Autodesk Inventor part; units mm, degrees
ref_plane "Arbeitsebene1" through (0, 5.7, 0) normal (0, 1, 0) x (1, 0, 0)
ref_plane "YZ Plane" through (0, 0, 0) normal (1, 0, 0) x (0, 1, 0)
ref_plane "XZ Plane" through (0, 0, 0) normal (0, 1, 0) x (-1, 0, 0)
sketch "Skizze2" plane through (0, 0, 0) normal (0, 1, 0) x (-1, 0, 0)
  line L0 (0, 0) -> (2.4, 0)
  line L1 (2.4, 0) -> (2.4, -5)
  line L2 (2.4, -5) -> (0, -5)
  line L3 (0, -5) -> (0, 0)
  dimension "d0" = 2.4
  dimension "d1" = 5
extrude "Extrusion1" add sketch "Skizze2" along normal blind 6.3
sketch "Skizze3" plane through (0, 0, 0) normal (0, -1, 0) x (1, 0, 0)
  line L0 (-0.9, -3.47) -> (-1.5, -3.47)
  line L1 (-1.5, -3.47) -> (-1.5, -4.07)
  line L2 (-1.5, -4.07) -> (-0.9, -4.07)
  line L3 (-0.9, -4.07) -> (-0.9, -3.47)
  line L4 (-0.9, -0.93) -> (-1.5, -0.93)
  line L5 (-1.5, -0.93) -> (-1.5, -1.53)
  line L6 (-1.5, -1.53) -> (-0.9, -1.53)
  line L7 (-0.9, -1.53) -> (-0.9, -0.93)
  line L8 (-2.4, -5) -> (0, -5)
  line L9 (-2.4, 0) -> (-2.4, -5)
  point P0 (0, 0)
  dimension "d4" = 0.6
  dimension "d5" = 0.6
  dimension "d6" = 0.6
  dimension "d7" = 0.6
  dimension "d8" = 2.54
  dimension "d9" = 0.93
  dimension "d10" = 0.9
  dimension "d11" = 0.9
sketch "Skizze5" plane through (0, 0, 0) normal (0, -1, 0) x (1, 0, 0)
  line L0 (-0.5, -0.5) -> (-1.9, -0.5)
  line L1 (-1.9, -0.5) -> (-1.9, -4.5)
  line L2 (-1.9, -4.5) -> (-0.5, -4.5)
  line L3 (-0.5, -4.5) -> (-0.5, -0.5)
  line L4 (-2.4, 0) -> (-2.4, -5)
  line L5 (0, -5) -> (-2.4, -5)
  point P0 (0, 0)
  dimension "d15" = 1.4
  dimension "d16" = 4
  dimension "d17" = 0.5
  dimension "d18" = 0.5
extrude "Extrusion2" cut sketch "Skizze5" against normal blind 0.2
extrude "Extrusion3" cut sketch "Skizze3" against normal blind 6
ref_plane "Arbeitsebene1" through (0, 5.7, 0) normal (0, 1, 0) x (1, 0, 0)
sketch "Skizze6" plane through (0, 5.7, 0) normal (0, 1, 0) x (1, 0, 0)
  line L0 (1, -1) -> (-3, -1)
  line L1 (-3, -1) -> (-3, 6)
  line L2 (-3, 6) -> (1, 6)
  line L3 (1, 6) -> (1, -1)
  line L4 (-0.1, 4.9) -> (-2.3, 4.9)
  line L5 (-2.3, 4.9) -> (-2.3, 0.1)
  line L6 (-2.3, 0.1) -> (-0.1, 0.1)
  line L7 (-0.1, 0.1) -> (-0.1, 4.9)
  line L8 (0, 5) -> (-2.4, 5)
  line L9 (0, 0) -> (0, 5)
  line L10 (0, 0) -> (-2.4, 0)
  line L11 (-2.4, 5) -> (-2.4, 0)
  dimension "d24" = 0.1
  dimension "d25" = 0.1
  dimension "d26" = 0.1
  dimension "d27" = 0.1
extrude "Extrusion5" cut sketch "Skizze6" against normal blind 0.6 contours L0 L1 L2 L3 | L9 L10 L11 L8
sketch "Skizze7" plane through (0, 0.2, 0) normal (0, -1, 0) x (1, 0, 0)
  line L0 (-0.5, -2.004) -> (-1.5, -2.004)
  line L1 (-1.5, -2.004) -> (-1.5, -2.996)
  line L2 (-1.5, -2.996) -> (-0.5, -2.996)
  line L3 (-0.5, -2.996) -> (-0.5, -2.004)
  line L4 (-1.5, -3.47) -> (-0.9, -3.47)
  line L5 (-0.9, -1.53) -> (-1.5, -1.53)
  line L6 (-0.5, -0.5) -> (-0.5, -4.5)
  line L7 (-1.5, -1.53) -> (-1.5, -0.93)
  line L8 (-1.5, -2.004) -> (-1.217, -2.004)
  line L9 (-1.217, -2.004) -> (-1.217, -1.53)
  line L10 (-1.217, -1.53) -> (-1.5, -1.53)
  line L11 (-1.5, -1.53) -> (-1.5, -2.004)
  line L12 (-1.5, -3.47) -> (-0.9, -3.47)
  line L13 (-1.5, -2.996) -> (-1.217, -2.996)
  line L14 (-1.217, -2.996) -> (-1.217, -3.47)
  line L15 (-1.217, -3.47) -> (-1.5, -3.47)
  line L16 (-1.5, -3.47) -> (-1.5, -2.996)
  point P0 (0, 0)
  dimension "d32" = 0.474
  dimension "d33" = 0.474
  dimension "d34" = 0.283
  dimension "d35" = 0.283
extrude "Extrusion6" cut sketch "Skizze7" against normal up to surface (5.8 mm away)
properties part number "Jumper"
Check sheet for the modelled part. Datum: model origin and axes. Units: mm. A direction names the side the tool comes from. Round coordinates to 2 decimals unless told otherwise and drop trailing zeros. Order: outer loops, then holes, each group sorted by start corner. A loop starts at its lowest first (then second) coordinate and runs counter-clockwise, first axis right, second up. Notation, with made-up numbers: (50, -26) - (83, -26) arc R17 ccw to (83, -17) - close; hole circle Ø2 at (33, 71.5). An arc over 180 degrees is marked (long way). Answer as CSV lines item,"result". Start each with the question number.
1) Section check D-D (y = 5.25). Record the cut outline in (x, z), then the cut area to 3 significant figures.
2) Section check B-B (x = -1). Record the cut outline in (y, z).
3) Scan lines: probe 1 along X at (y, z) = (1.75, -1.95); probe 2 along Z at (x, y) = (-1.15, 2); probe 3 along X at (y, z) = (5.5, -1.7). Record each from-to range of solid material in increasing order.
4) Tool access check on faces 4 (the face through (-1.5, 3, -2)), 5 (the face through (-2.4, 3, -2)). Record the directions out of +Z, -Z, +X, -X, +Y, -Y that give a thin tool (end or side, any length) a straight path to the whole face; none if there is none.
5) Section check C-C (z = -3.15). Record the cut outline in (x, y).
6) Depth check by flat-ended pin: pin 1 (0.7 mm diameter, centred on x = -1, z = -2, fed in from -Y). Enter the tip coordinate at first touch or a pass-through.
7) Section check A-A (y = 1.5). Record the cut outline in (x, z).
8) Draft check along Y on faces 1 (the face through (-1, 6.3, -2)), 2 (the face through (-1.7, 0.2, -2.5)), 3 (the face through (-1, 3, 0)). Enter one of: +Y half, -Y half, draft (parallel to the pull), parting line (faces both ways), or undercut.
Determined:
1,outline,"(-2.3, -4.9) - (-0.1, -4.9) - (-0.1, -0.1) - (-2.3, -0.1) - close; hole (-1.5, -4.07) - (-0.9, -4.07) - (-0.9, -3.47) - (-1.22, -3.47) - (-1.22, -3) - (-0.5, -3) - (-0.5, -2) - (-1.22, -2) - (-1.22, -1.53) - (-0.9, -1.53) - (-0.9, -0.93) - (-1.5, -0.93) - close"
1,area,"8.58 mm^2"
2,outline,"(0, -5) - (5.1, -5) - (5.1, -4.9) - (5.7, -4.9) - (5.7, -5) - (6.3, -5) - (6.3, 0) - (5.7, 0) - (5.7, -0.1) - (5.1, -0.1) - (5.1, 0) - (0, 0) - (0, -0.5) - (0.2, -0.5) - (0.2, -0.93) - (6, -0.93) - (6, -1.53) - (0.2, -1.53) - (0.2, -2) - (6, -2) - (6, -3) - (0.2, -3) - (0.2, -3.47) - (6, -3.47) - (6, -4.07) - (0.2, -4.07) - (0.2, -4.5) - (0, -4.5) - close"
3,probe 1,"-2.4 to -1.5, -1.22 to 0"
3,probe 2,"-5 to -4.07, -3.47 to -3, -2 to -1.53, -0.93 to 0"
3,probe 3,"-2.3 to -1.5, -1.22 to -0.1"
4,face 4,"-Y"
4,face 5,"+Z, -Z, -X, +Y, -Y"
5,outline,"(-2.4, 0) - (-1.9, 0) - (-1.9, 0.2) - (-1.5, 0.2) - (-1.5, 6) - (-1.22, 6) - (-1.22, 0.2) - (-0.5, 0.2) - (-0.5, 0) - (0, 0) - (0, 5.1) - (-0.1, 5.1) - (-0.1, 5.7) - (0, 5.7) - (0, 6.3) - (-2.4, 6.3) - (-2.4, 5.7) - (-2.3, 5.7) - (-2.3, 5.1) - (-2.4, 5.1) - close"
6,pin 1,"y = 0.2"
7,outline,"(-2.4, -5) - (0, -5) - (0, 0) - (-2.4, 0) - close; hole (-1.5, -4.07) - (-0.9, -4.07) - (-0.9, -3.47) - (-1.22, -3.47) - (-1.22, -3) - (-0.5, -3) - (-0.5, -2) - (-1.22, -2) - (-1.22, -1.53) - (-0.9, -1.53) - (-0.9, -0.93) - (-1.5, -0.93) - close"
8,face 1,"+Y half"
8,face 2,"-Y half"
8,face 3,"draft"
